Drawing for the job (mm, zero at the part's lowest x, y, z). Give positions to 0.01 mm unless a question says otherwise; leave off trailing zeros. Write each loop counter-clockwise with the first axis right and the second up, starting at its lowest first coordinate (ties: lowest second). Pieces come first, ordered by that corner, then holes.
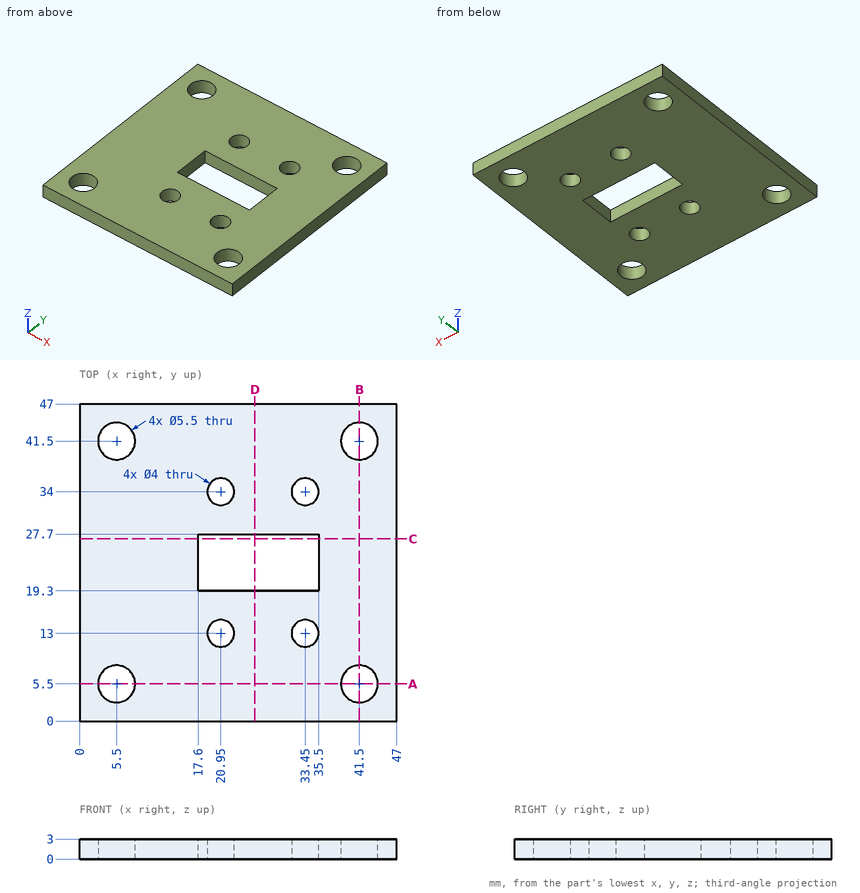
1. Slice it at A-A, the plane y = 5.5. Write the cut outline in (x, z), and give its area (3 significant figures).
Calculated:
outline: (0, 0) - (2.75, 0) - (2.75, 3) - (0, 3) - close; (8.25, 0) - (38.75, 0) - (38.75, 3) - (8.25, 3) - close; (44.25, 0) - (47, 0) - (47, 3) - (44.25, 3) - close
area: 108 mm2
2. Pin check, flat tip, straight feed: P1, Ø2.5, axis at x = 33.45, y = 34, coming from the +Z side. Stop position of the tip, or through.
Calculated:
P1: passes through
3. Slice it at D-D, the plane x = 26. Write the cut outline in (y, z), and give its area (3 significant figures).
Calculated:
outline: (0, 0) - (19.3, 0) - (19.3, 3) - (0, 3) - close; (27.7, 0) - (47, 0) - (47, 3) - (27.7, 3) - close
area: 116 mm2
4. Slice it at C-C, the plane y = 27. Write the cut outline in (x, z), and give its area (3 significant figures).
Calculated:
outline: (0, 0) - (17.6, 0) - (17.6, 3) - (0, 3) - close; (35.5, 0) - (47, 0) - (47, 3) - (35.5, 3) - close
area: 87.3 mm2
5. Probe probe 1 along Y at (x, z) = (41.5, 1.1); probe 2 along Y at (x, z) = (33.45, 1.3); probe 3 along Y at (x, z) = (35, 2.05). List the from-to ranges inside material, lowest first.
Calculated:
probe 1: y = 0 to 2.75, 8.25 to 38.75, 44.25 to 47
probe 2: y = 0 to 11, 15 to 19.3, 27.7 to 32, 36 to 47
probe 3: y = 0 to 11.74, 14.26 to 19.3, 27.7 to 32.74, 35.26 to 47
